Check sheet for the modelled part. Datum: model origin and axes. Units: mm. Give positions to 0.01 mm unless a question says otherwise; leave off trailing zeros. Loops run counter-clockwise (first coordinate to the right, second up) from the corner with the lowest first, then second, coordinate; pieces in that order, holes last. Notation, with made-up numbers: M -19,-36.75 L 0,-36.75 A29 ccw 0,-15.75 Z; hole C 55,12.5 d10. An arc over 180 degrees is marked long. One line per question, with ' | ' between items. Start each with the question number.
from build123d import *

# Parameters (mm, degrees)
SKETCH1_W           = 279.4
SKETCH1_H           = 88.9
BOSS_EXTRUDE1_DEPTH = 12.7
SKETCH2_R           = 2.1463
CUT_EXTRUDE1_DEPTH  = 38.1
CUT_EXTRUDE2_START  = -38.1
SKETCH3_R           = 2.1463
CUT_EXTRUDE2_DEPTH  = 38.1
SKETCH4_R           = 6.0071
CUT_EXTRUDE3_DEPTH  = 294.477188211
SKETCH5_R           = 2.38125
CUT_EXTRUDE4_DEPTH  = 294.477188211


with BuildPart() as part:
    # Sketch1 → Boss-Extrude1 (new body)
    with BuildSketch(Plane.XY):
        with Locations((139.7, 44.45)):
            Rectangle(SKETCH1_W, SKETCH1_H)
    extrude(amount=BOSS_EXTRUDE1_DEPTH)

    # Sketch2 → Cut-Extrude1 (cut)
    with BuildSketch(Plane(origin=(279.4, 0, 0), x_dir=(0, 0, -1), z_dir=(1, 0, 0))):
        with Locations((-6.35, 76.2)):
            Circle(SKETCH2_R)
        with Locations((-6.35, 12.7)):
            Circle(SKETCH2_R)
    extrude(amount=-CUT_EXTRUDE1_DEPTH, mode=Mode.SUBTRACT)

    # Sketch3 → Cut-Extrude2 (cut)
    with BuildSketch(Plane.ZY.offset(CUT_EXTRUDE2_START)):
        with Locations(Location((6.35, 76.2, 0), (0, 0, 180))):
            Circle(SKETCH3_R)
        with Locations(Location((6.35, 12.7, 0), (0, 0, 180))):
            Circle(SKETCH3_R)
    extrude(amount=CUT_EXTRUDE2_DEPTH, mode=Mode.SUBTRACT)

    # Sketch4 → Cut-Extrude3 (cut, through all)
    with BuildSketch(Plane(origin=(0, 0, 0), x_dir=(-1, 0, 0), z_dir=(0, 0, -1))):
        with Locations((-209.55, 31.75)):
            Circle(SKETCH4_R)
        with Locations((-139.7, 31.75)):
            Circle(SKETCH4_R)
        with Locations((-69.85, 31.75)):
            Circle(SKETCH4_R)
    extrude(amount=-CUT_EXTRUDE3_DEPTH, mode=Mode.SUBTRACT)

    # Sketch5 → Cut-Extrude4 (cut, through all)
    with BuildSketch(Plane.XY):
        with Locations((163.06165, 55.11165)):
            Circle(SKETCH5_R)
        with Locations((116.33835, 55.11165)):
            Circle(SKETCH5_R)
        with Locations((116.33835, 8.38835)):
            Circle(SKETCH5_R)
        with Locations((163.06165, 8.38835)):
            Circle(SKETCH5_R)
    extrude(amount=CUT_EXTRUDE4_DEPTH, mode=Mode.SUBTRACT)


solid = part.part
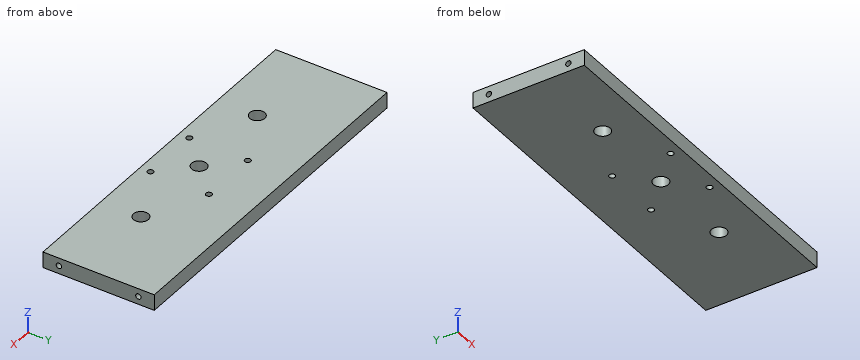
Q1. Cross-section at B-B (x = 209.55). Record the cut outline in (y, z).
Q2. Depth check by flat-ended pin: P1, Ø3, axis at x = 163.06, y = 55.11, coming from the -Z side; P2, Ø2, axis at y = 12.5, z = 5.5, coming from the -X side; P3, Ø2.5, axis at y = 76.2, z = 6.35, coming from the +X side. Enter the tip coordinate at first touch or a pass-through.
Q3. Cross-section at C-C (x = 19). Record the cut outline in (y, z).
Q4. Material ranges on probe 1 along Y at (x, z) = (15, 6.35); probe 2 along X at (y, z) = (32.5, 6.75); probe 3 along Y at (x, z) = (209.55, 3), recorded low to high. Write a range as from..to.
Q5. Cross-section at A-A (y = 31.75). Record the cut outline in (x, z), and give its area (3 significant figures).
Q6. Cross-section at D-D (z = 6.35). Record the cut outline in (x, y), and give its area (3 significant figures).
Solved:
1) outline: M 0,0 L 25.74,0 L 25.74,12.7 L 0,12.7 Z; M 37.76,0 L 88.9,0 L 88.9,12.7 L 37.76,12.7 Z
2) P1: passes through | P2: stops at x = 38.1 | P3: stops at x = 241.3
3) outline: M 0,0 L 88.9,0 L 88.9,12.7 L 0,12.7 Z; hole C 12.7,6.35 d4.29; hole C 76.2,6.35 d4.29
4) probe 1: y = 0..10.55, 14.85..74.05, 78.35..88.9 | probe 2: x = 0..63.89, 75.81..133.74, 145.66..203.59, 215.51..279.4 | probe 3: y = 0..25.74, 37.76..88.9
5) outline: M 0,0 L 63.84,0 L 63.84,12.7 L 0,12.7 Z; M 75.86,0 L 133.69,0 L 133.69,12.7 L 75.86,12.7 Z; M 145.71,0 L 203.54,0 L 203.54,12.7 L 145.71,12.7 Z; M 215.56,0 L 279.4,0 L 279.4,12.7 L 215.56,12.7 Z | area: 3,090 mm²
6) outline: M 0,0 L 279.4,0 L 279.4,10.55 L 241.3,10.55 L 241.3,14.85 L 279.4,14.85 L 279.4,74.05 L 241.3,74.05 L 241.3,78.35 L 279.4,78.35 L 279.4,88.9 L 0,88.9 L 0,78.35 L 38.1,78.35 L 38.1,74.05 L 0,74.05 L 0,14.85 L 38.1,14.85 L 38.1,10.55 L 0,10.55 Z; hole C 69.85,31.75 d12.01; hole C 116.34,8.39 d4.76; hole C 116.34,55.11 d4.76; hole C 139.7,31.75 d12.01; hole C 163.06,8.39 d4.76; hole C 163.06,55.11 d4.76; hole C 209.55,31.75 d12.01 | area: 23,800 mm²
